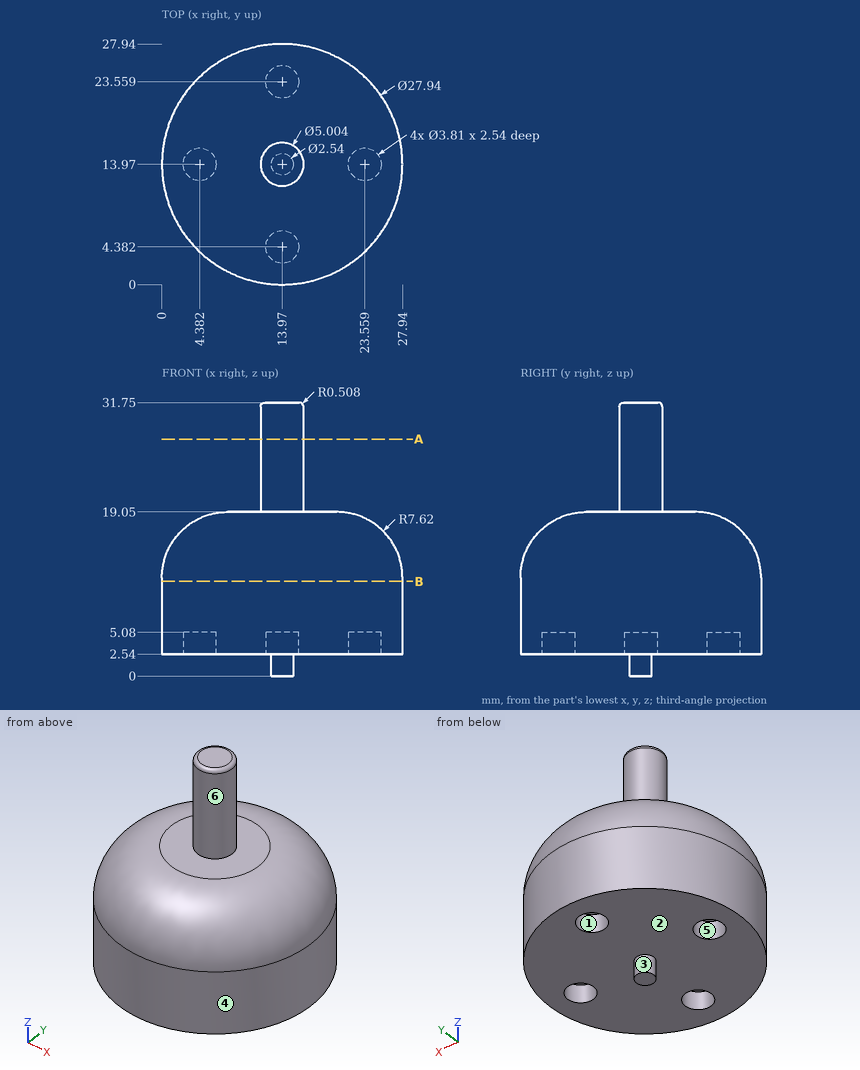
Geometry check sheet. Reference: drawing and pictorial views, mm from the part's lowest x, y, z. A direction names the side the tool comes from. Coordinates: 2 decimals unless noted, no trailing zeros. Write each loop counter-clockwise with the first axis right and the second up, starting at its lowest first coordinate (ties: lowest second). Pieces come first, ordered by that corner, then holes. Notation, with made-up numbers: (4.25, -29) -> (8.25, -29) arc R12 ccw to (8.25, -24) -> close; hole circle Ø1 at (84.5, -1.5). An arc over 180 degrees is marked (long way). Use a Markdown table: item, result.
1. Scan lines: line 1 along Y through (x, z) = (13.97, 3.6); line 2 along Y through (x, z) = (5.5, 4.5); line 3 along Y through (x, z) = (4.75, 3) (1 decimal). Record each from-to range of solid material in increasing order.
Reported:
| item | result |
|---|---|
| line 1 | y = 0 to 2.48, 6.29 to 21.65, 25.46 to 27.94 |
| line 2 | y = 2.86 to 12.43, 15.51 to 25.08 |
| line 3 | y = 3.5 to 12.1, 15.8 to 24.5 |
2. Release check for a two-part mould opening along Y. For the marked faces 1, 2 and 3 record: pulls with the +Y half, pulls with the -Y half, needs draft (parallel to the pull), parting line crosses it, or undercut.
Reported:
| item | result |
|---|---|
| face 1 | undercut |
| face 2 | needs draft |
| face 3 | parting line crosses it |
3. Sectioned sample at A-A (z = 27.5). Enter the section's corners in (x, y).
Reported:
| item | result |
|---|---|
| outline | circle Ø5 at (13.97, 13.97) |
4. Go/stop test with flat-tipped pins: pin 1 Ø5 at (x, y) = (23.56, 13.97) entering from +Z; pin 2 Ø4 at (x, y) = (23.5, 14) entering from -Z; pin 3 Ø3 at (x, y) = (13.97, 23.56) entering from +Z. Record where each tip stops, or that it passes through.
Reported:
| item | result |
|---|---|
| pin 1 | stops at z = 19.01 |
| pin 2 | stops at z = 2.54 |
| pin 3 | stops at z = 18.85 |
5. Tool access check on the marked faces 4, 5 and 6. Record the directions out of +Z, -Z, +X, -X, +Y, -Y that give a thin tool (end or side, any length) a straight path to the whole face; none if there is none.
Reported:
| item | result |
|---|---|
| face 4 | +Z, -Z |
| face 5 | -Z |
| face 6 | +Z |
6. Sectioned sample at B-B (z = 11). Enter the section's corners in (x, y), plus the area to 3 significant figures.
Reported:
| item | result |
|---|---|
| outline | circle Ø27.94 at (13.97, 13.97) |
| area | 613 mm2 |
